Autodesk Inventor part; units mm, degrees
ref_plane "YZ Plane" through (0, 0, 0) normal (1, 0, 0) x (0, 1, 0)
ref_plane "XZ Plane" through (0, 0, 0) normal (0, 1, 0) x (-1, 0, 0)
ref_plane "XY Plane" through (0, 0, 0) normal (0, 0, 1) x (1, 0, 0)
sketch "Sketch1" plane through (0, 0, 0) normal (0, 0, 1) x (1, 0, 0)
  line L0 (-11, 43) -> (13, 43)
  line L1 (13, 43) -> (13, -43)
  line L2 (13, -43) -> (-11, -43)
  line L3 (-11, -43) -> (-11, 43)
  point P0 (0, 0)
  dimension "d0" = 24
  dimension "d1" = 86
  dimension "d2" = 43
  dimension "d3" = 11
extrude "Extrusion1" add sketch "Sketch1" along normal blind 2
sketch "Sketch2" plane through (0, 0, 2) normal (0, 0, 1) x (1, 0, 0)
  circle A0 centre (-5.8, 0) radius 3.25
  line L0 (13, -43) -> (13, 43)
  point P0 (0, 0)
  dimension "d6" = 6.5
  dimension "d7" = 18.8
extrude "Extrusion2" cut sketch "Sketch2" against normal blind 2
sketch "Sketch3" plane through (0, 0, 2) normal (0, 0, 1) x (1, 0, 0)
  line L0 (13, 43) -> (-11, 43)
  line L1 (13, -43) -> (13, 43)
  line L2 (-11, 43) -> (13, 43)
  line L3 (13, 43) -> (13, 41)
  line L4 (13, 41) -> (-11, 41)
  line L5 (-11, 41) -> (-11, 43)
  line L6 (-11, -43) -> (13, -43)
  line L7 (13, -43) -> (13, -41)
  line L8 (13, -41) -> (-11, -41)
  line L9 (-11, -41) -> (-11, -43)
  line L10 (13, -41) -> (11, -41)
  line L11 (11, -41) -> (11, 41)
  line L12 (11, 41) -> (13, 41)
  line L13 (13, 41) -> (13, -41)
  line L14 (-11, 43) -> (-11, -43)
  line L15 (-11, -43) -> (13, -43)
  point P0 (0, 0)
  dimension "d10" = 2
  dimension "d11" = 2
  dimension "d12" = 2
extrude "Extrusion3" cut sketch "Sketch3" against normal blind 2 contours L1 L4 L5 L0 | L1 L8 L11 L4 | L1 L6 L9 L8
properties part number "top-1"
Geometry: final body of the model. Coordinates: model frame, mm. Round coordinates to 2 decimals unless told otherwise and drop trailing zeros. Order: outer loops, then holes, each group sorted by start corner. A loop starts at its lowest first (then second) coordinate and runs counter-clockwise, first axis right, second up. Notation, with made-up numbers: (-10, 82) - (6, 82) arc R21 cw to (6, 118) - close; hole circle Ø6 at (37, 37.5). An arc over 180 degrees is marked (long way). Use CSV: the item, a comma, the result in double quotes. Start each with the question number.
Q1. Section query B-B (y = 0). Return loops of the section in (x, z), and give its area (3 significant figures).
Q2. Material intervals for line 1 along Y through (x, z) = (-5.8, 0.75); line 2 along Y through (x, z) = (-7, 0.35); line 3 along X through (y, z) = (-1, 0.1), sorted ascending. Write a range as from..to.
Q3. Mould query, pull axis X, two halves, no side actions, for faces 1 (the face through (-11, -1, 1)), 2 (the face through (0, 1, 2)), 3 (the face through (11, -1, 1)), 4 (the face through (-9.047, 0.143, 1.014)). Classes: +X half, -X half, draft (parallel to the pull), parting line (faces both ways), or undercut.
Q4. Section query A-A (x = -5.8). Return loops of the section in (y, z), and give its area (3 significant figures).
Q5. Section query C-C (z = 0.6). Return loops of the section in (x, y), and give its area (3 significant figures).
Result set:
1,outline,"(-11, 0) - (-9.05, 0) - (-9.05, 2) - (-11, 2) - close; (-2.55, 0) - (11, 0) - (11, 2) - (-2.55, 2) - close"
1,area,"31.0 mm2"
2,line 1,"y = -41..-3.25, 3.25..41"
2,line 2,"y = -41..-3.02, 3.02..41"
2,line 3,"x = -11..-8.89, -2.71..11"
3,face 1,"-X half"
3,face 2,"draft"
3,face 3,"+X half"
3,face 4,"undercut"
4,outline,"(-41, 0) - (-3.25, 0) - (-3.25, 2) - (-41, 2) - close; (3.25, 0) - (41, 0) - (41, 2) - (3.25, 2) - close"
4,area,"151 mm2"
5,outline,"(-11, -41) - (11, -41) - (11, 41) - (-11, 41) - close; hole circle Ø6.5 at (-5.8, 0)"
5,area,"1,770 mm2"
